from build123d import *

# Parameters (mm, degrees)
F2_SIZE = 8.99999


# Not quite as in the source:
# - a fillet or chamfer is up to 0.001 mm smaller than in the source, because OpenCascade refuses the exact size


with BuildPart() as f1:
    # F0 (on Right) → F1 (revolve)
    with BuildSketch(Plane.YZ):
        Polygon((-37.8479540345, 16.603627705), (-37.8479540345, 76.603627705), (-46.8479540345, 76.603627705), (-46.8479540345, 8.603627705), (-37.8479540345, 8.603627705), (-37.8479540345, 0.603627705), (-2.8479540345, 0.603627705), (-2.8479540345, 8.603627705), (-27.8479540345, 8.603627705), (-27.8479540345, 16.603627705), align=None)
    revolve(axis=Axis((0, -2.8479540345, 4.603627705), (0, 0, 1)))

    # F2 (size 9 in the source; OpenCascade refuses exactly that, so slightly less here)
    f2_edges = [f1.edges().sort_by_distance(p)[0] for p in [
        (0, 32.152046, 76.603628),
    ]]
    chamfer(f2_edges, length=F2_SIZE)


solid = f1.part
Geometry check sheet. Reference: the model listing, model coordinates, mm. A direction names the side the tool comes from. Give positions to 0.01 mm unless a question says otherwise; leave off trailing zeros. Order: outer loops, then holes, each group sorted by start corner. A loop starts at its lowest first (then second) coordinate and runs counter-clockwise, first axis right, second up. Notation, with made-up numbers: (35.25, 18) - (91.25, 18) arc R16 cw to (91.25, 48) - close; hole circle Ø1 at (12.5, -1.75). An arc over 180 degrees is marked (long way). Use one line per item in the form item = value.
1) Material ranges on probe 1 along Z at (x, y) = (-10.5, -6.5); probe 2 along Z at (x, y) = (11.5, -34.5); probe 3 along Y at (x, z) = (-28.5, 72), recorded low to high. Write a range as from..to.
Working result:
probe_1 = 0.6..8.6
probe_2 = 0.6..16.6
probe_3 = -36.37..-30.05, 24.35..30.67
2) Access from +Z, -Z, +X, -X, +Y, -Y to the whole of each face (thin tool, end or side, straight path). Record for faces 1 (the face through (-19, 27, 8.604)), 2 (the face through (0, -3, 8.604)).
Working result:
face_1 = -Z
face_2 = +Z
3) Depth check by flat-ended pin: pin 1 Ø10 at (y, z) = (29, 52.5) entering from +X; pin 2 Ø3 at (x, y) = (24.5, -23.5) entering from +Z; pin 3 Ø5 at (x, z) = (26, 47) entering from -Y. Enter the tip coordinate at first touch or a pass-through.
Working result:
pin_1 = 34.86
pin_2 = 16.6
pin_3 = -40.05
4) Sectioned sample at C-C (z = 20). Record the boundary of the cut face in (x, y), and give its area (3 significant figures).
Working result:
outline = circle Ø88 at (0, -2.85); hole circle Ø70 at (0, -2.85)
area = 2,230 mm^2
5) Sectioned sample at B-B (z = 6). Record the boundary of the cut face in (x, y), and give its area (3 significant figures).
Working result:
outline = circle Ø70 at (0, -2.85)
area = 3,850 mm^2
6) Draft check along X on faces 3 (the face through (-39.036, -23.151, 42.128)), 4 (the face through (7.509, -26.694, 12.66)), 5 (the face through (0, -2, 0.604)). Enter one of: released by +X, released by -X, zero draft, split by the parting line, or undercut.
Working result:
face_3 = split by the parting line
face_4 = undercut
face_5 = zero draft
